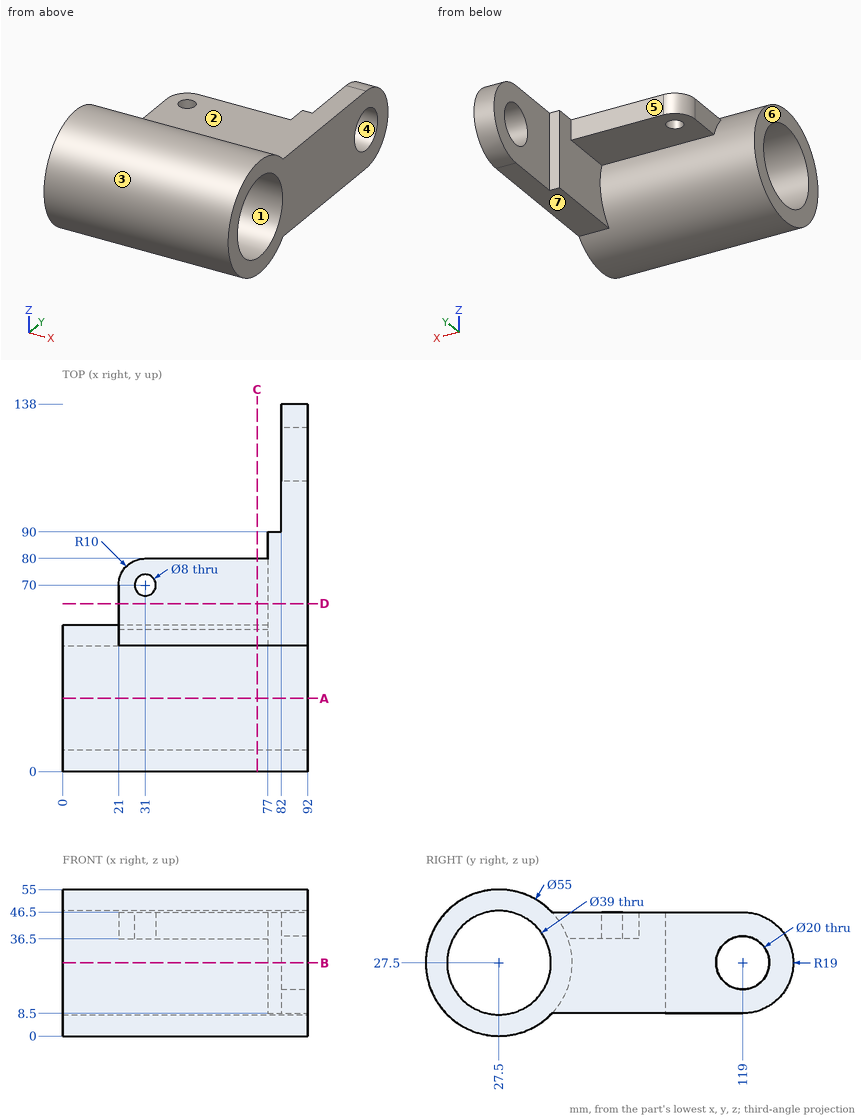
Geometry: see drawing. Coordinates: mm, zero at the bounding-box minimum. A direction names the side the tool comes from. Round coordinates to 2 decimals unless told otherwise and drop trailing zeros. Write each loop counter-clockwise with the first axis right and the second up, starting at its lowest first coordinate (ties: lowest second). Pieces come first, ordered by that corner, then holes.
Item 1: Section query B-B (z = 27.5). Return loops of the section in (x, y), plus the area to 3 significant figures.
Item 2: Pin query (flat end, axial travel): P1, Ø5, axis at x = 43.5, z = 35, coming from the -Y side; P2, Ø4, axis at x = 57.5, z = 40, coming from the +Y side; P3, Ø8, axis at x = 57.5, z = 29.5, coming from the +Y side. Return the tip coordinate at first contact, or that it passes through.
Item 3: Mould query, pull axis Y, two halves, no side actions, for the marked faces 1, 2, 3 and 4. Classes: +Y half, -Y half, draft (parallel to the pull), parting line (faces both ways), or undercut.
Item 4: Section query A-A (y = 27.5). Return loops of the section in (x, z).
Item 5: Set-up query: the marked faces 5, 6 and 7. Return all of +Z, -Z, +X, -X, +Y, -Y with unobstructed straight access to the full face (end or side cutting, diameter ignored); none if empty.
Item 6: Material intervals for L1, parallel to Z at x = 88.75, y = 119; L2, parallel to Y at x = 31, z = 44; L3, parallel to Z at x = 35, y = 27, sorted ascending.
Item 7: Section query D-D (y = 63). Return loops of the section in (x, z), plus the area to 3 significant figures.
Item 8: Section query C-C (x = 73). Return loops of the section in (y, z).
Completed:
1. outline: (0, 0) - (92, 0) - (92, 8) - (0, 8) - close; (0, 47) - (92, 47) - (92, 109) - (82, 109) - (82, 90) - (77, 90) - (77, 55) - (0, 55) - close; (82, 129) - (92, 129) - (92, 138) - (82, 138) - close
1. area: 2,280 mm2
2. P1: stops at y = 0.46
2. P2: stops at y = 80
2. P3: stops at y = 55
3. face 1: undercut
3. face 2: draft
3. face 3: parting line
3. face 4: undercut
4. outline: (0, 0) - (92, 0) - (92, 8) - (0, 8) - close; (0, 47) - (92, 47) - (92, 55) - (0, 55) - close
5. face 5: +Z, -Z, -X, +Y
5. face 6: +Z, -Z, -X, +Y, -Y
5. face 7: -Z, +X, -X, +Y
6. L1: z = 8.5 to 17.5, 37.5 to 46.5
6. L2: y = 5.5 to 17.11, 37.89 to 66, 74 to 80
6. L3: z = 0 to 8.01, 46.99 to 55
7. outline: (21, 36.5) - (77, 36.5) - (77, 8.5) - (92, 8.5) - (92, 46.5) - (21, 46.5) - close
7. area: 1,130 mm2
8. outline: (47.38, 46.5) arc R27.5 ccw (long way) to (53.49, 36.5) - (80, 36.5) - (80, 46.5) - close; hole circle Ø39 at (27.5, 27.5)
